```python
from build123d import *

# Parameters (mm, degrees)
BOSS_EXTRUDE1_DEPTH = 3.8
SKETCH1_3_W         = 20.9
SKETCH1_3_H         = 12.6
BOSS_EXTRUDE2_DEPTH = 4
SKETCH3_R           = 2.5
BOSS_EXTRUDE4_DEPTH = 5
SKETCH5_R           = 1.65
CUT_EXTRUDE1_DEPTH  = 4


with BuildPart() as part:
    # Sketch1 → Boss-Extrude1 (new body)
    with BuildSketch(Plane(origin=(0, 0, 0), x_dir=(1, 0, 0), z_dir=(0, 1, 0))):
        Polygon((22.9, 14.6), (-2, 14.6), (-2, 0), (0, 0), (0, 12.6), (20.9, 12.6), (20.9, 0), (22.9, 0), align=None)
    extrude(amount=BOSS_EXTRUDE1_DEPTH)

    # Sketch1<3> → Boss-Extrude2 (add)
    with BuildSketch(Plane(origin=(0, 0, 0), x_dir=(1, 0, 0), z_dir=(0, 1, 0))):
        with Locations((10.45, 6.3)):
            Rectangle(SKETCH1_3_W, SKETCH1_3_H)
        Polygon((22.9, 14.6), (-2, 14.6), (-2, 0), (0, 0), (0, 12.6), (20.9, 12.6), (20.9, 0), (22.9, 0), align=None)
    extrude(amount=-BOSS_EXTRUDE2_DEPTH)

    # Sketch3 → Boss-Extrude4 (add)
    with BuildSketch(Plane.XZ.offset(4)):
        with Locations(Location((5.45, -7.3, 0), (0, 0, 90))):
            Circle(SKETCH3_R)
        with Locations(Location((15.45, -7.3, 0), (0, 0, 90))):
            Circle(SKETCH3_R)
    extrude(amount=BOSS_EXTRUDE4_DEPTH)

    # Sketch5 → Cut-Extrude1 (cut)
    with BuildSketch(Plane(origin=(0, 0, 0), x_dir=(1, 0, 0), z_dir=(0, 1, 0))):
        with Locations(Location((2.67, 10.55, 0), (0, 0, 270))):
            Circle(SKETCH5_R)
        with Locations(Location((18.23, 10.55, 0), (0, 0, 270))):
            Circle(SKETCH5_R)
    extrude(amount=-CUT_EXTRUDE1_DEPTH, mode=Mode.SUBTRACT)


solid = part.part
```
Here's how the part is built. I have some questions about the finished solid (model axes, mm). A direction names the side the tool comes from. Give positions to 0.01 mm unless a question says otherwise; leave off trailing zeros. Order: outer loops, then holes, each group sorted by start corner. A loop starts at its lowest first (then second) coordinate and runs counter-clockwise, first axis right, second up. Notation, with made-up numbers: M -37.5,87.25 L 10.5,87.25 A22 cw 10.5,123.25 Z; hole C -30.5,-26 d5. An arc over 180 degrees is marked long. Use a Markdown table: item, result. Add a question column.
1. If we mould it in two halves opening along X, with no side actions, what happens to faces 4 (the cylindrical face through (6.41, -6.46, -4.99)), 5 (the flat face through (11, 0, -14.6)), 6 (the flat face through (22.9, 0, -7))? For each: +X half, -X half, draft (parallel to the pull), parting line (faces both ways), or undercut.
2. Suppose I cut it at D-D (y = -8). List the corners of the cut face in (x, z) for me.
3. For pin 1 Ø4 at (y, z) = (-6.5, -9.5) entering from +X; pin 2 Ø1.5 at (x, y) = (7.5, -5.5) entering from -Z; pin 3 Ø6 at (x, z) = (10.5, -12.5) entering from -Y, each with a flat end and sliding along its axis, tell me the tip position at first contact or that it passes through.
4. I need wall thicknesses on probe 1 along X at (y, z) = (-1.7, -10.55); probe 2 along X at (y, z) = (-7.25, -7.25); probe 3 along Z at (x, y) = (19.5, 0.75). Which ranges of each line are inside material? Lowest first, please. Write a range as from..to.
5. Suppose I cut it at A-A (z = -10.55). List the corners of the cut face in (x, y) for me, and give its area (3 significant figures).
6. On a 3-axis mill with a long thin cutter (end or side, diameter ignored), from which of +Z, -Z, +X, -X, +Y, -Y can I reach the whole of each face in a straight line? I mean faces 1 (the flat face through (10, -4, -7)), 2 (the flat face through (10, 0, -6)), 3 (the flat face through (10, -1, 0)). Say none if no direction works.
7. Suppose I cut it at B-B (x = 2.67). List the corners of the cut face in (y, z) for me.
8. Suppose I cut it at C-C (y = -3.5). List the corners of the cut face in (x, z) for me.
Results list:
| question | item | result |
|---|---|---|
| 1 | face 4 | undercut |
| 1 | face 5 | draft |
| 1 | face 6 | +X half |
| 2 | outline | C 5.45,-7.3 d5; C 15.45,-7.3 d5 |
| 3 | pin 1 | stops at x = 17.94 |
| 3 | pin 2 | stops at z = -9.44 |
| 3 | pin 3 | stops at y = -4 |
| 4 | probe 1 | x = -2..1.02, 4.32..16.58, 19.88..22.9 |
| 4 | probe 2 | x = 2.95..7.95, 12.95..17.95 |
| 4 | probe 3 | z = -14.6..-12.6 |
| 5 | outline | M -2,-4 L 1.02,-4 L 1.02,0 L 0,0 L 0,3.8 L -2,3.8 Z; M 4.32,-4 L 16.58,-4 L 16.58,0 L 4.32,0 Z; M 19.88,-4 L 22.9,-4 L 22.9,3.8 L 20.9,3.8 L 20.9,0 L 19.88,0 Z |
| 5 | area | 88.4 mm² |
| 6 | face 1 | -Y |
| 6 | face 2 | +Z, +Y |
| 6 | face 3 | +Z, +X, -X, +Y, -Y |
| 7 | outline | M -4,-14.6 L 3.8,-14.6 L 3.8,-12.6 L 0,-12.6 L 0,-12.2 L -4,-12.2 Z; M -4,-8.9 L 0,-8.9 L 0,0 L -4,0 Z |
| 8 | outline | M -2,-14.6 L 22.9,-14.6 L 22.9,0 L -2,0 Z; hole C 2.67,-10.55 d3.3; hole C 18.23,-10.55 d3.3 |
